Autodesk Fusion 360 part; units mm, degrees
sketch "Sketch1" plane through (0, 0, 0) normal (0, 0, 1) x (1, 0, 0)
  line L0 (-28, 37) -> (62, 37)
  line L1 (62, 37) -> (62, 18)
  line L2 (62, 18) -> (-28, 18)
  line L3 (-28, 18) -> (-28, 37)
  dimension "d1" = 90
  dimension "d2" = 19
extrude "Extrude1" add sketch "Sketch1" along normal blind 6
fillet "Fillet1" radius 7 3 edges at (62, 37, 3) (62, 18, 3) (-28, 18, 3)
fillet "Fillet2" radius 7 1 edges at (-28, 37, 3)
sketch "Sketch2" plane through (0, 0, 6) normal (0, 0, 1) x (-1, 0, 0)
  arc A0 (21, -37) -> (28, -30) centre (21, -30) ccw
  line L0 (28, -30) -> (28, -25)
  arc A1 (28, -25) -> (21, -18) centre (21, -25) ccw
  line L1 (21, -18) -> (-55, -18)
  arc A2 (-55, -18) -> (-62, -25) centre (-55, -25) ccw
  line L2 (-62, -25) -> (-62, -30)
  arc A3 (-62, -30) -> (-55, -37) centre (-55, -30) ccw
  line L3 (-55, -37) -> (21, -37)
ref_plane "WorkPlane1" through (17, 27.5, 6) normal (0, 0, 1) x (-1, 0, 0)
sketch "Sketch3" plane through (0, 0, 6) normal (0, 0, 1) x (1, 0, 0)
  line L0 (17, 37) -> (17, 18)
  circle A0 centre (-8, 27.5) radius 8.9
  circle A1 centre (42, 27.5) radius 8.9
  circle A2 centre (-8, 27.5) radius 3.65
  circle A3 centre (42, 27.5) radius 3.65
  dimension "d13" = 17.8
  dimension "d14" = 17.8
  dimension "d15" = 7.3
  dimension "d16" = 7.3
extrude "Extrude2" cut sketch "Sketch3" against normal blind 7 contours A2 | A3
extrude "Extrude3" cut sketch "Sketch3" against normal blind 3
sketch "Sketch4" plane through (0, 0, 0) normal (0, 0, 1) x (1, 0, 0)
  line L0 (-21, 37) -> (55, 37)
  line L1 (55, 37) -> (55, 39)
  line L2 (55, 39) -> (-21, 39)
  line L3 (-21, 39) -> (-21, 37)
  dimension "d21" = 76
  dimension "d22" = 2
extrude "Extrude4" add sketch "Sketch4" along normal blind 13
ref_plane "WorkPlane2" through (-21, 38, 6.5) normal (-1, 0, 0) x (0, -1, 0)
sketch "Sketch5" plane through (-21, 0, 0) normal (-1, 0, 0) x (0, -1, 0)
  line L0 (-39, 13) -> (-49, 13)
  line L1 (-49, 13) -> (-49, 12)
  line L2 (-39, 13) -> (-39, 11)
  line L3 (-49, 12.5) -> (-39, 11)
  dimension "d26" = 10
  dimension "d27" = 1
extrude "Extrude5" add sketch "Sketch5" against normal blind 76
sketch "Sketch6" plane through (-21, 0, 0) normal (-1, 0, 0) x (0, -1, 0)
  line L0 (-39, 0) -> (-37, 0)
  line L1 (-37, 0) -> (-37, 6)
  line L2 (-37, 6) -> (-37, 13)
  line L3 (-37, 13) -> (-49, 13)
  line L4 (-49, 13) -> (-49, 12.5)
  line L5 (-49, 12.5) -> (-39, 11)
  line L6 (-39, 11) -> (-39, 0)
  line L7 (-39, 7.5) -> (-49, 7.5)
  line L8 (-49, 7.5) -> (-49, 6.3428)
  line L9 (-49, 6.3428) -> (-39, 3.3342)
  line L10 (-39, 7.5) -> (-39, 3.3342)
  dimension "d34" = 10
extrude "Extrude6" add sketch "Sketch6" against normal blind 76 contours L6 L7 L8 L9 L10
Can you work these out from the model? Positions are in its coordinate system, mm. A direction names the side the tool comes from. Coordinates: 2 decimals unless noted, no trailing zeros. Loops run counter-clockwise (first coordinate to the right, second up) from the corner with the lowest first, then second, coordinate; pieces in that order, holes last.
1) Which directions (+Z, -Z, +X, -X, +Y, -Y) give clear straight access to the entire face, cutting with the end or side of a thin tool? Please do faces 1 (the flat face through (46, 28, 3)), 2 (the flat face through (16, 37, 9)), 3 (the flat face through (16, 43, 13)).
2) Imagine slicing it at D-D on z = 8.75. List the corners of the cut face in (x, y) for me, plus the area to 3 significant figures.
3) Imagine slicing it at A-A on x = -8. List the corners of the cut face in (y, z) for me, plus the area to 3 significant figures.
4) Imagine slicing it at B-B on y = 27.5. List the corners of the cut face in (x, z) for me.
5) Imagine slicing it at C-C on x = 18. List the corners of the cut face in (y, z) for me, plus the area to 3 significant figures.
6) I need wall thicknesses on probe 1 along Y at (x, z) = (-8, 2.15); probe 2 along X at (y, z) = (21, 4); probe 3 along Z at (x, y) = (17, 25). Which ranges of each line are inside material? Lowest first, please.
7) For pin 1 (2 mm diameter, centred on x = 23, z = 8, fed in from -Y); pin 2 (11.5 mm diameter, centred on x = 42, y = 27.5, fed in from +Z); pin 3 (6 mm diameter, centred on y = 44.5, z = 8.5, fed in from -X), each with a flat end and sliding along its axis, tell me the tip position at first contact or that it passes through.
8) Thinking about a two-plate mould opening in X: for faces 4 (the cylindrical face through (34.94, 22.08, 4.52)), 5 (the cylindrical face through (60, 34.9, 3)), 6 (the flat face through (-21, 42, 7)), 7 (the flat face through (-4, 28, 3)), which applies, pulls with the +X half, pulls with the -X half, needs draft (parallel to the pull), parting line crosses it, or undercut?
Completed:
1. face 1: +Z
1. face 2: +Z, +X, -X, -Y
1. face 3: +Z, +X, -X, +Y, -Y
2. outline: (-21, 37) - (55, 37) - (55, 39) - (-21, 39) - close
2. area: 152 mm2
3. outline: (18, 0) - (23.85, 0) - (23.85, 3) - (18.6, 3) - (18.6, 6) - (18, 6) - close; (31.15, 0) - (39, 0) - (39, 3.33) - (49, 6.34) - (49, 7.5) - (39, 7.5) - (39, 11) - (49, 12.5) - (49, 13) - (37, 13) - (37, 6) - (36.4, 6) - (36.4, 3) - (31.15, 3) - close
3. area: 104 mm2
4. outline: (-28, 0) - (-11.65, 0) - (-11.65, 3) - (-16.9, 3) - (-16.9, 6) - (-28, 6) - close; (-4.35, 0) - (38.35, 0) - (38.35, 3) - (33.1, 3) - (33.1, 6) - (0.9, 6) - (0.9, 3) - (-4.35, 3) - close; (45.65, 0) - (62, 0) - (62, 6) - (50.9, 6) - (50.9, 3) - (45.65, 3) - close
5. outline: (18, 0) - (39, 0) - (39, 3.33) - (49, 6.34) - (49, 7.5) - (39, 7.5) - (39, 11) - (49, 12.5) - (49, 13) - (37, 13) - (37, 6) - (18, 6) - close
5. area: 179 mm2
6. probe 1: y = 18 to 23.85, 31.15 to 39
6. probe 2: x = -26.74 to -14.08, -1.92 to 35.92, 48.08 to 60.74
6. probe 3: z = 0 to 6
7. pin 1: stops at y = 37
7. pin 2: stops at z = 3
7. pin 3: stops at x = -21
8. face 4: undercut
8. face 5: pulls with the +X half
8. face 6: pulls with the -X half
8. face 7: undercut
